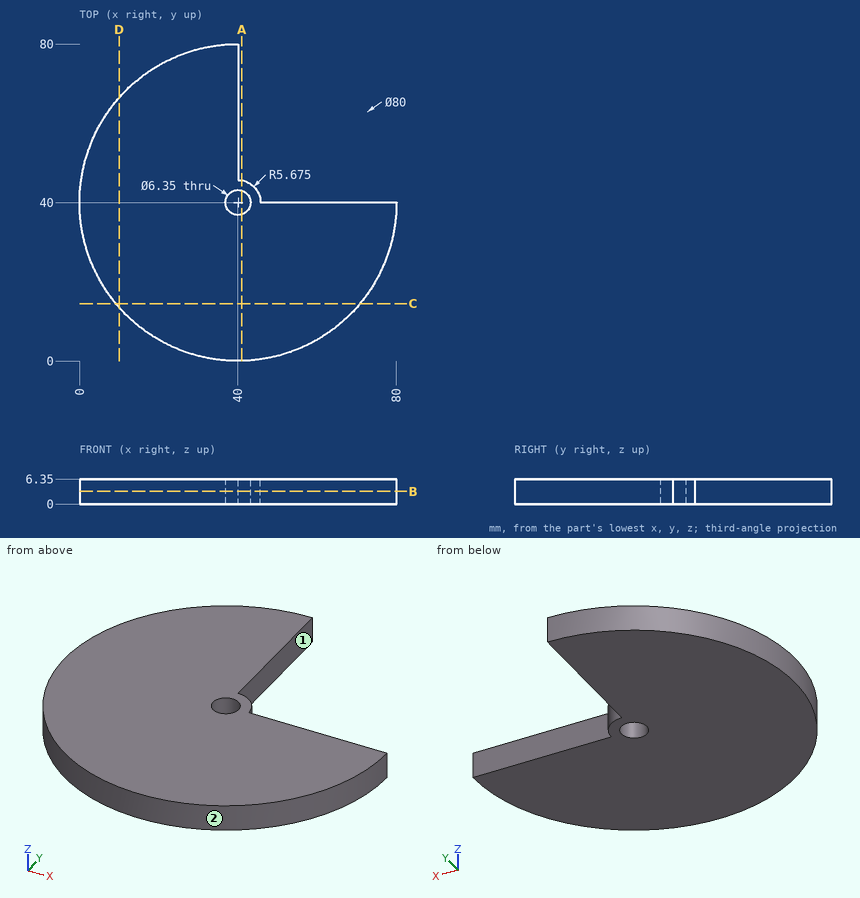
Design review of the part shown in the three views and the two pictorial views. Dimensions are in mm from the part's minimum x, y and z. A direction names the side the tool comes from. Round coordinates to 2 decimals unless told otherwise and drop trailing zeros. Loops run counter-clockwise (first coordinate to the right, second up) from the corner with the lowest first, then second, coordinate; pieces in that order, holes last.
1) Consider section A-A on x = 41. State the section outline as (y, z) points.
Values follow:
outline: (0.01, 0) - (36.99, 0) - (36.99, 6.35) - (0.01, 6.35) - close; (43.01, 0) - (45.59, 0) - (45.59, 6.35) - (43.01, 6.35) - close
2) Tool access review of the marked faces 1 and 2: name each direction out of +Z, -Z, +X, -X, +Y, -Y from which nothing blocks a thin tool from reaching the whole face with its end or side.
Values follow:
face 1: +Z, -Z, +X, +Y
face 2: +Z, -Z
3) Consider section D-D on x = 10. State the section outline as (y, z) points.
Values follow:
outline: (13.54, 0) - (66.46, 0) - (66.46, 6.35) - (13.54, 6.35) - close
4) Consider section C-C on y = 14.5. State the section outline as (x, z) points, then the cut area to 3 significant figures.
Values follow:
outline: (9.18, 0) - (70.82, 0) - (70.82, 6.35) - (9.18, 6.35) - close
area: 391 mm2
5) Clearance check with flat-ended pins moving along their axes: P1, Ø3, axis at y = 9, z = 3.5, coming from the -X side; P2, Ø1.5, axis at y = 19.5, z = 3, coming from the -X side; P3, Ø5, axis at x = 68, y = 10.5, coming from the -Z side; P4, Ø1.5, axis at y = 11.5, z = 5, coming from the +X side. State where each tip first meets the part, or that it passes through.
Values follow:
P1: stops at x = 12.99
P2: stops at x = 5.22
P3: stops at z = 0
P4: stops at x = 68.81
6) Consider section B-B on z = 3.25. State the section outline as (x, y) points (3 decimals), then the cut area to 3 significant figures.
Values follow:
outline: (40, 45.675) - (40, 80) arc R40 ccw (long way) to (80, 40) - (45.675, 40) arc R5.675 ccw to start; hole circle Ø6.35 at (40, 40)
area: 3,760 mm2
7) Wall thickness on line 1 along X through (y, z) = (47, 2.75); line 2 along X through (y, z) = (27.5, 2.5); line 3 along Y through (x, z) = (60, 6.25): over which ranges is each line inside the solid? List them lowest first.
Values follow:
line 1: x = 0.62 to 40
line 2: x = 2 to 78
line 3: y = 5.36 to 40
